```python
from build123d import *

# Parameters (mm, degrees)
SKETCH1_R           = 1.15
SKETCH1_R_2         = 6.05
SKETCH1_R_3         = 2.85
BOSS_EXTRUDE1_DEPTH = 1.5
SKETCH3_R           = 6.05
SKETCH3_R_2         = 5.781920351
BOSS_EXTRUDE6_DEPTH = 10.1


with BuildPart() as part:
    # Sketch1 → Boss-Extrude1 (new body)
    # profile 1 of 3: a face of its own
    with BuildSketch(Plane(origin=(0, 0, 0), x_dir=(1, 0, 0), z_dir=(0, 1, 0))):
        with BuildLine():
            ThreePointArc((-13.51764198, -2.768029891), (-8.071510009, -3.409034399), (-2.923037011, -5.297013747))
            ThreePointArc((-2.923037011, -5.297013747), (-6.05, 0), (-2.923037011, 5.297013747))
            ThreePointArc((-2.923037011, 5.297013747), (-8.078843984, 3.456352976), (-13.51764198, 2.831970109))
            ThreePointArc((-13.51764198, 2.831970109), (-16.31764198, 0.031970109), (-13.51764198, -2.768029891))
        make_face()
        with Locations(Location((-13.51764198, 0.031970109, 0), (0, 0, 270))):
            Circle(SKETCH1_R, mode=Mode.SUBTRACT)
    # profile 2 of 3: a face of its own
    with BuildSketch(Plane(origin=(0, 0, 0), x_dir=(1, 0, 0), z_dir=(0, 1, 0))):
        Circle(SKETCH1_R_2)
        with Locations(Location((0, 0, 0), (0, 0, 270))):
            Circle(SKETCH1_R_3, mode=Mode.SUBTRACT)
    # profile 3 of 3: a face of its own
    with BuildSketch(Plane(origin=(0, 0, 0), x_dir=(1, 0, 0), z_dir=(0, 1, 0))):
        with BuildLine():
            ThreePointArc((2.923037011, -5.297013747), (8.053384371, -3.409091417), (13.48235802, -2.768029891))
            ThreePointArc((13.48235802, -2.768029891), (16.28235802, 0.031970109), (13.48235802, 2.831970109))
            ThreePointArc((13.48235802, 2.831970109), (8.060741556, 3.456405922), (2.923037011, 5.297013747))
            ThreePointArc((2.923037011, 5.297013747), (5.209936368, 3.07555898), (6.05, 0))
            ThreePointArc((6.05, 0), (5.209936368, -3.07555898), (2.923037011, -5.297013747))
        make_face()
        with Locations(Location((13.48235802, 0.031970109, 0), (0, 0, 270))):
            Circle(SKETCH1_R, mode=Mode.SUBTRACT)
    extrude(amount=BOSS_EXTRUDE1_DEPTH)

    # Sketch3 → Boss-Extrude6 (add)
    with BuildSketch(Plane(origin=(0, 0, 0), x_dir=(1, 0, 0), z_dir=(0, 1, 0))):
        with Locations(Location((0, 0, 0), (0, 0, 118.891114763))):
            Circle(SKETCH3_R)
        with Locations(Location((0, 0, 0), (0, 0, 270))):
            Circle(SKETCH3_R_2, mode=Mode.SUBTRACT)
    extrude(amount=BOSS_EXTRUDE6_DEPTH)


solid = part.part
```
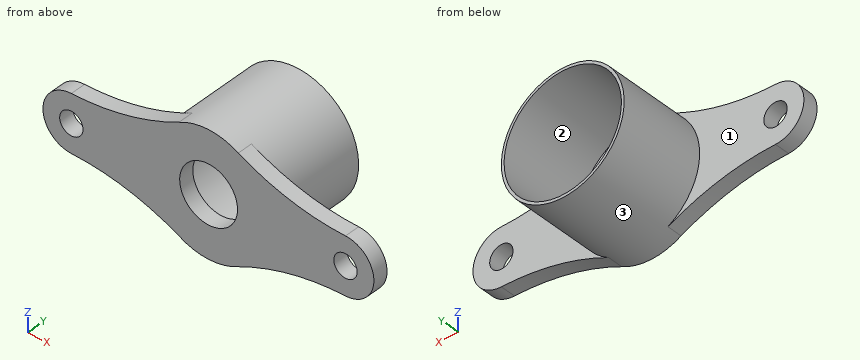
Source: CAD feature listing. Evaluate the final solid. Frame: model axes, mm. Face numbers are marked on the shaded views. Give positions to 0.01 mm unless a question says otherwise; leave off trailing zeros. Write each loop counter-clockwise with the first axis right and the second up, starting at its lowest first coordinate (ties: lowest second). Pieces come first, ordered by that corner, then holes.
1. Section query B-B (z = 0). Return the cut outline in (x, y), then the cut area to 3 significant figures.
2. Pull-direction query (Z, two-part tool) for the marked faces 1, 2 and 3; classes: +Z half, -Z half, draft (parallel to the pull), parting line (faces both ways), or undercut.
3. First-contact query: pin 1 (2 mm diameter, centred on x = 13.48, z = -0.03, fed in from +Y); pin 2 (6 mm diameter, centred on x = 4, y = 5, fed in from -Z); pin 3 (5.5 mm diameter, centred on x = -9.5, z = 0.5, fed in from +Y); pin 4 (3 mm diameter, centred on x = 4.5, y = 9, fed in from -Z). Flat tips, straight axial feed; report the tip coordinate or a pass-through.
4. Section query D-D (x = -14). Return the cut outline in (y, z).
5. Material intervals for line 1 along Z through (x, y) = (0, 6); line 2 along Y through (x, z) = (-1.5, -4.5), sorted ascending.
6. Section query A-A (x = 0). Return the cut outline in (y, z).
7. Section query C-C (y = 6.75). Return the cut outline in (x, z).
Output values:
1. outline: (-16.32, 0) - (-14.67, 0) - (-14.67, 1.5) - (-16.32, 1.5) - close; (-12.37, 0) - (-2.85, 0) - (-2.85, 1.5) - (-5.78, 1.5) - (-5.78, 10.1) - (-6.05, 10.1) - (-6.05, 1.5) - (-12.37, 1.5) - close; (2.85, 0) - (12.33, 0) - (12.33, 1.5) - (6.05, 1.5) - (6.05, 10.1) - (5.78, 10.1) - (5.78, 1.5) - (2.85, 1.5) - close; (14.63, 0) - (16.28, 0) - (16.28, 1.5) - (14.63, 1.5) - close
1. area: 38.1 mm2
2. face 1: draft
2. face 2: undercut
2. face 3: parting line
3. pin 1: passes through
3. pin 2: stops at z = -5.97
3. pin 3: stops at y = 1.5
3. pin 4: stops at z = -5.25
4. outline: (0, -2.79) - (1.5, -2.79) - (1.5, -1.08) - (0, -1.08) - close; (0, 1.01) - (1.5, 1.01) - (1.5, 2.73) - (0, 2.73) - close
5. line 1: z = -6.05 to -5.78, 5.78 to 6.05
5. line 2: y = 0 to 1.5
6. outline: (0, -6.05) - (10.1, -6.05) - (10.1, -5.78) - (1.5, -5.78) - (1.5, -2.85) - (0, -2.85) - close; (0, 2.85) - (1.5, 2.85) - (1.5, 5.78) - (10.1, 5.78) - (10.1, 6.05) - (0, 6.05) - close
7. outline: circle Ø12.1 at (0, 0); hole circle Ø11.56 at (0, 0)
